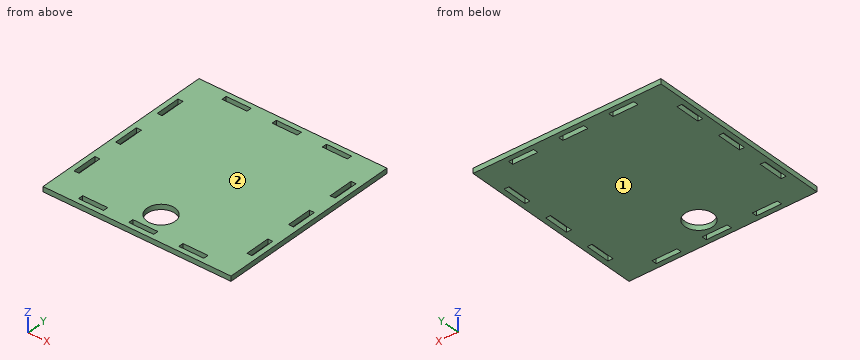
```python
from build123d import *

# Parameters (mm, degrees)
F0_W     = 150
F0_H     = 150
F0_R     = 11.15
F1_DEPTH = 4


with BuildPart() as f1:
    # F0 (on Top) → F1 (new body)
    with BuildSketch(Plane.XY):
        Rectangle(F0_W, F0_H)
        Polygon((-30, -71), (-40, -71), (-50, -71), (-50, -67), (-40, -67), (-30, -67), align=None, mode=Mode.SUBTRACT)
        Polygon((-71, -30), (-67, -30), (-67, -50), (-71, -50), (-71, -40), align=None, mode=Mode.SUBTRACT)
        Polygon((-10, -71), (-10, -67), (0, -67), (10, -67), (10, -71), (0, -71), align=None, mode=Mode.SUBTRACT)
        with Locations((0, -51.85)):
            Circle(F0_R, mode=Mode.SUBTRACT)
        Polygon((50, -71), (40, -71), (30, -71), (30, -67), (40, -67), (50, -67), align=None, mode=Mode.SUBTRACT)
        Polygon((71, -50), (67, -50), (67, -30), (71, -30), (71, -40), align=None, mode=Mode.SUBTRACT)
        Polygon((-71, -10), (-71, 0), (-71, 10), (-67, 10), (-67, 0), (-67, -10), align=None, mode=Mode.SUBTRACT)
        Polygon((-71, 50), (-67, 50), (-67, 30), (-71, 30), (-71, 40), align=None, mode=Mode.SUBTRACT)
        Polygon((-30, 71), (-30, 67), (-40, 67), (-50, 67), (-50, 71), (-40, 71), align=None, mode=Mode.SUBTRACT)
        Polygon((71, 0), (71, -10), (67, -10), (67, 10), (71, 10), align=None, mode=Mode.SUBTRACT)
        Polygon((-10, 71), (0, 71), (10, 71), (10, 67), (0, 67), (-10, 67), align=None, mode=Mode.SUBTRACT)
        Polygon((71, 30), (67, 30), (67, 50), (71, 50), (71, 40), align=None, mode=Mode.SUBTRACT)
        Polygon((30, 71), (40, 71), (50, 71), (50, 67), (40, 67), (30, 67), align=None, mode=Mode.SUBTRACT)
    extrude(amount=F1_DEPTH)


solid = f1.part
```
Here's how the part is built. I have some questions about the finished solid (model axes, mm). Face numbers are marked on the shaded views. Coordinates: 2 decimals unless noted, no trailing zeros. Write each loop counter-clockwise with the first axis right and the second up, starting at its lowest first coordinate (ties: lowest second). Pieces come first, ordered by that corner, then holes. Notation, with made-up numbers: M 27.25,15.25 L 63.25,15.25 A16 cw 63.25,44.25 Z; hole C 8,-24.5 d4. An arc over 180 degrees is marked long. Answer as CSV lines item,"result". Start each with the question number.
Q1. Suppose I cut it at D-D, the plane z = 1.45. State how many separate pieces and enclosed holes the cut face has, then the cut area to 3 significant figures.
Q2. I need wall thicknesses on probe 1 along Y at (x, z) = (0, 1.45); probe 2 along Y at (x, z) = (-37.5, 3.2); probe 3 along Y at (x, z) = (-68.5, 1.95). Which ranges of each line are inside material? Lowest first, please. Write a range as [from, to].
Q3. Suppose I cut it at B-B, the plane x = 0. List the corners of the cut face in (y, z) for me, then the cut area to 3 significant figures.
Q4. If we mould it in two halves opening along Z, with no side actions, what happens to the marked faces 1 and 2? For each: pulls with the +Z half, pulls with the -Z half, needs draft (parallel to the pull), parting line crosses it, or undercut.
Q5. Suppose I cut it at C-C, the plane y = 40. List the corners of the cut face in (x, z) for me, then the cut area to 3 significant figures.
Q6. Suppose I cut it at A-A, the plane y = -51.85. List the corners of the cut face in (x, z) for me.
Entries:
1,separate pieces,"1"
1,enclosed holes,"13"
1,area,"21,100 mm²"
2,probe 1,"y = [-75, -71], [-67, -63], [-40.7, 67], [71, 75]"
2,probe 2,"y = [-75, -71], [-67, 67], [71, 75]"
2,probe 3,"y = [-75, -50], [-30, -10], [10, 30], [50, 75]"
3,outline,"M -75,0 L -71,0 L -71,4 L -75,4 Z; M -67,0 L -63,0 L -63,4 L -67,4 Z; M -40.7,0 L 67,0 L 67,4 L -40.7,4 Z; M 71,0 L 75,0 L 75,4 L 71,4 Z"
3,area,"479 mm²"
4,face 1,"pulls with the -Z half"
4,face 2,"pulls with the +Z half"
5,outline,"M -75,0 L -71,0 L -71,4 L -75,4 Z; M -67,0 L 67,0 L 67,4 L -67,4 Z; M 71,0 L 75,0 L 75,4 L 71,4 Z"
5,area,"568 mm²"
6,outline,"M -75,0 L -11.15,0 L -11.15,4 L -75,4 Z; M 11.15,0 L 75,0 L 75,4 L 11.15,4 Z"
